Build history of the part. All positions in model axes, mm. A direction names the side the tool comes from. Give positions to 0.01 mm unless a question says otherwise; leave off trailing zeros. Loops run counter-clockwise (first coordinate to the right, second up) from the corner with the lowest first, then second, coordinate; pieces in that order, holes last. Notation, with made-up numbers: (45.5, 0.25) -> (95.5, 0.25) arc R22 ccw to (95.5, 11.25) -> close; hole circle Ø1 at (72, -34). An arc over 180 degrees is marked (long way). Answer as a JSON object with one key per item and string values. Group by question number.
Q1. Drop flat-ended pins along their axis: pin 1 (1.2 mm diameter, centred on y = 2, z = 2, fed in from +X); pin 2 (2 mm diameter, centred on x = 59, z = 3, fed in from +Y); pin 3 (1.2 mm diameter, centred on x = 203.5, z = 2.5, fed in from -Y). Give the stop position or say it passes through.
Q2. Band-saw the part on A-A, the plane x = 123.5. Write the cut outline in (y, z).
Q3. Band-saw the part on B-B, the plane x = 263. Write the cut outline in (y, z).
Q4. Band-saw the part on C-C, the plane z = 1.35. Count the separate pieces of the cut face and the enclosed holes in it, plus the area to 3 significant figures.
Q5. Tool access for faces 4 (the flat face through (157, 7, 0)), 5 (the flat face through (263.008, -4.467, 1.972)), 6 (the flat face through (164.311, -18.136, 1.972)): list every direction of +Z, -Z, +X, -X, +Y, -Y with a clear straight run to the whole face (end or side of a thin tool).
Q6. Wall check: probe 1 along Y at (x, z) = (57.5, 0.5); probe 2 along X at (y, z) = (14, 3.8); probe 3 along Y at (x, z) = (30, 2.05). Give the ranges that are in metal, low to high. Write a range as from..to.
Q7. Two-plate mould, pull along X, no slides. Class faces 1 (the flat face through (-1.31, 21.99, 1.97)), 2 (the cylindrical face through (328.582, 4.832, 1.972)), 3 (the flat face through (164.826, 2.476, 1.972)): pulls with the +X half, pulls with the -X half, needs draft (parallel to the pull), parting line crosses it, or undercut.
from build123d import *

# Parameters (mm, degrees)
SKETCH_1_R          = 9.7
SKETCH_1_R_2        = 5.2
SKETCH_1_R_3        = 2
EXTRUDE_1_DEPTH     = 4
CUT_EXTRUDE_1_DEPTH = 10


with BuildPart() as part:
    # 草图1 → 凸台-拉伸1 (new body)
    with BuildSketch(Plane.XY):
        with BuildLine():
            Line((-9.85, 17.060700455), (7.470508076, 27.060700455))
            Line((7.470508076, 27.060700455), (289.624667154, 27.060700455))
            ThreePointArc((289.624667154, 27.060700455), (328.694852344, 4.11311011), (297.66555963, -28.905888469))
            Line((297.66555963, -28.905888469), (27.170508076, -7.060700455))
            Line((27.170508076, -7.060700455), (9.85, -17.060700455))
            ThreePointArc((9.85, -17.060700455), (-17.060700455, -9.85), (-9.85, 17.060700455))
        make_face()
        Circle(SKETCH_1_R, mode=Mode.SUBTRACT)
        with Locations((300, 0)):
            Circle(SKETCH_1_R_2, mode=Mode.SUBTRACT)
        with Locations((319, 0)):
            Circle(SKETCH_1_R_3, mode=Mode.SUBTRACT)
        with Locations((313.435028843, -13.435028843)):
            Circle(SKETCH_1_R_3, mode=Mode.SUBTRACT)
        with Locations((300, -19)):
            Circle(SKETCH_1_R_3, mode=Mode.SUBTRACT)
        with Locations((286.564971157, -13.435028843)):
            Circle(SKETCH_1_R_3, mode=Mode.SUBTRACT)
        with Locations((281, 0)):
            Circle(SKETCH_1_R_3, mode=Mode.SUBTRACT)
        with Locations((286.564971157, 13.435028843)):
            Circle(SKETCH_1_R_3, mode=Mode.SUBTRACT)
        with Locations((300, 19)):
            Circle(SKETCH_1_R_3, mode=Mode.SUBTRACT)
        with Locations((313.435028843, 13.435028843)):
            Circle(SKETCH_1_R_3, mode=Mode.SUBTRACT)
        with Locations((250, 20)):
            Circle(SKETCH_1_R_3, mode=Mode.SUBTRACT)
        with Locations((195, 20)):
            Circle(SKETCH_1_R_3, mode=Mode.SUBTRACT)
        with Locations((140, 20)):
            Circle(SKETCH_1_R_3, mode=Mode.SUBTRACT)
        with Locations((85, 20)):
            Circle(SKETCH_1_R_3, mode=Mode.SUBTRACT)
        with Locations((30, 20)):
            Circle(SKETCH_1_R_3, mode=Mode.SUBTRACT)
        with Locations(Location((250, -20, 0), (0, 0, 180))):
            Circle(SKETCH_1_R_3, mode=Mode.SUBTRACT)
        with Locations((167.5, -13.337297667)):
            Circle(SKETCH_1_R_3, mode=Mode.SUBTRACT)
        with Locations((57.5, -4.453694555)):
            Circle(SKETCH_1_R_3, mode=Mode.SUBTRACT)
    extrude(amount=EXTRUDE_1_DEPTH)

    # 草图2 → 切除-拉伸1 (cut)
    with BuildSketch(Plane(origin=(0, 0, 0), x_dir=(-1, 0, 0), z_dir=(0, 0, -1))):
        with BuildLine():
            Line((-137.197603441, 10.82531174), (-106.043706264, 1.591034337))
            ThreePointArc((-106.043706264, 1.591034337), (-105.333274422, 0.528665045), (-106.247395472, -0.364489265))
            Line((-106.247395472, -0.364489265), (-146.939942745, -3.650820533))
            ThreePointArc((-146.939942745, -3.650820533), (-147.907056702, -3.116572023), (-147.791851116, -2.017727835))
            Line((-147.791851116, -2.017727835), (-137.197603441, 10.82531174))
        make_face()
        with BuildLine():
            Line((-242, 12), (-159.091058121, 12))
            ThreePointArc((-159.091058121, 12), (-158.186531194, 11.426416508), (-158.319647694, 10.363662077))
            Line((-158.319647694, 10.363662077), (-171.517559676, -5.635709572))
            Line((-171.517559676, -5.635709572), (-242, -11.327873446))
            Line((-242, -11.327873446), (-242, 12))
        make_face()
        with BuildLine():
            Line((-77.967218715, 12), (-53.665101582, 12))
            ThreePointArc((-53.665101582, 12), (-52.730413268, 11.355468359), (-53.000597339, 10.252715509))
            Line((-53.000597339, 10.252715509), (-59.49167188, 4.480688084))
            Line((-59.49167188, 4.480688084), (-78.251405867, 10.041231173))
            ThreePointArc((-78.251405867, 10.041231173), (-78.956857242, 11.14358129), (-77.967218715, 12))
        make_face()
        with BuildLine():
            Line((-268.630020148, 0.840296648), (-257.54212687, 7.993776182))
            ThreePointArc((-257.54212687, 7.993776182), (-256.52152684, 8.031581712), (-256, 7.153479534))
            Line((-256, 7.153479534), (-256, -7.153479534))
            ThreePointArc((-256, -7.153479534), (-256.52152684, -8.031581712), (-257.54212687, -7.993776182))
            Line((-257.54212687, -7.993776182), (-268.630020148, -0.840296648))
            ThreePointArc((-268.630020148, -0.840296648), (-269.087893278, 0), (-268.630020148, 0.840296648))
        make_face()
        with BuildLine():
            Line((-19.631707517, 7.078552885), (-29.56189752, 13.698679554))
            Line((-29.56189752, 13.698679554), (-40.860283753, 3.651869157))
            ThreePointArc((-40.860283753, 3.651869157), (-41.116034111, 2.513264507), (-40.118555254, 1.907570918))
            Line((-40.118555254, 1.907570918), (-20.586659398, 3.4204248))
            ThreePointArc((-20.586659398, 3.4204248), (-18.805958358, 4.909282805), (-19.631707517, 7.078552885))
        make_face()
    extrude(amount=-CUT_EXTRUDE_1_DEPTH, mode=Mode.SUBTRACT)


solid = part.part
Worked answers:
{
 "1": {"pin 1": "x = 328.96", "pin 2": "y = 27.06", "pin 3": "y = -21.35"},
 "2": {"outline": "(-14.84, 0) -> (-1.76, 0) -> (-1.76, 4) -> (-14.84, 4) -> close; (6.77, 0) -> (27.06, 0) -> (27.06, 4) -> (6.77, 4) -> close"},
 "3": {"outline": "(-26.11, 0) -> (-4.47, 0) -> (-4.47, 4) -> (-26.11, 4) -> close; (4.47, 0) -> (27.06, 0) -> (27.06, 4) -> (4.47, 4) -> close"},
 "4": {"separate pieces": "1", "enclosed holes": "23", "area": "12,500 mm2"},
 "5": {"face 4": "-Z, +X, -X, +Y, -Y", "face 5": "+Z, -Z", "face 6": "+Z, -Z, -Y"},
 "6": {"probe 1": "-9.51..-6.45, -2.45..6.25, 12..27.06", "probe 2": "-13.86..284.65, 288.48..311.52, 315.35..325.38", "probe 3": "-7.29..2.69, 13.31..18, 22..27.06"},
 "7": {"face 1": "pulls with the -X half", "face 2": "parting line crosses it", "face 3": "undercut"}
}
